Check sheet for the modelled part. Datum: model origin and axes. Units: mm. A direction names the side the tool comes from. Give positions to 0.01 mm unless a question says otherwise; leave off trailing zeros. Order: outer loops, then holes, each group sorted by start corner. A loop starts at its lowest first (then second) coordinate and runs counter-clockwise, first axis right, second up.
```python
from build123d import *

# Parameters (mm, degrees)
IZIM1_R                     = 6.55
Y_KSEKLIK_EKSTR_ZYON1_DEPTH = 1.6
IZIM2_R                     = 1.5
KES_EKSTR_ZYON1_DEPTH       = 1.6


with BuildPart() as part:
    # Çizim1 → Yükseklik-Ekstrüzyon1 (new body)
    with BuildSketch(Plane.XY):
        with BuildLine():
            Line((51.878679656, -0.878679656), (62.901413512, -11.901413512))
            ThreePointArc((62.901413512, -11.901413512), (63.179114484, -12.782168471), (62.616924992, -13.51482808))
            Line((62.616924992, -13.51482808), (61.615557944, -13.981773203))
            ThreePointArc((61.615557944, -13.981773203), (60.959512838, -14.047839782), (60.404952381, -13.691156907))
            ThreePointArc((60.404952381, -13.691156907), (53.799180994, -16.856750014), (61.123557768, -16.753308252))
            ThreePointArc((61.123557768, -16.753308252), (61.318334892, -16.334489822), (61.680554911, -16.047882666))
            Line((61.680554911, -16.047882666), (63.577381738, -15.16337779))
            ThreePointArc((63.577381738, -15.16337779), (64.537299608, -15.226294131), (65, -16.069685577))
            Line((65, -16.069685577), (65, -66.030314423))
            ThreePointArc((65, -66.030314423), (64.537299608, -66.873705869), (63.577381738, -66.93662221))
            Line((63.577381738, -66.93662221), (61.680554911, -66.052117334))
            ThreePointArc((61.680554911, -66.052117334), (61.318334892, -65.765510178), (61.123557768, -65.346691748))
            ThreePointArc((61.123557768, -65.346691748), (53.799180994, -65.243249986), (60.404952381, -68.408843093))
            ThreePointArc((60.404952381, -68.408843093), (60.959512838, -68.052160218), (61.615557944, -68.118226797))
            Line((61.615557944, -68.118226797), (62.616924992, -68.58517192))
            ThreePointArc((62.616924992, -68.58517192), (63.179114484, -69.317831529), (62.901413512, -70.198586488))
            Line((62.901413512, -70.198586488), (51.878679656, -81.221320344))
            ThreePointArc((51.878679656, -81.221320344), (50.90540961, -81.871638598), (49.757359313, -82.1))
            Line((49.757359313, -82.1), (34.45, -82.1))
            ThreePointArc((34.45, -82.1), (33.742893219, -81.807106781), (33.45, -81.1))
            Line((33.45, -81.1), (33.45, -80.681281566))
            ThreePointArc((33.45, -80.681281566), (33.610200525, -80.138384852), (34.039473684, -79.769432815))
            ThreePointArc((34.039473684, -79.769432815), (32.5, -72.6), (30.960526316, -79.769432815))
            ThreePointArc((30.960526316, -79.769432815), (31.389799475, -80.138384852), (31.55, -80.681281566))
            Line((31.55, -80.681281566), (31.55, -81.1))
            ThreePointArc((31.55, -81.1), (31.257106781, -81.807106781), (30.55, -82.1))
            Line((30.55, -82.1), (15.242640687, -82.1))
            ThreePointArc((15.242640687, -82.1), (14.09459039, -81.871638598), (13.121320344, -81.221320344))
            Line((13.121320344, -81.221320344), (2.098586488, -70.198586488))
            ThreePointArc((2.098586488, -70.198586488), (1.820885516, -69.317831529), (2.383075008, -68.58517192))
            Line((2.383075008, -68.58517192), (3.384442056, -68.118226797))
            ThreePointArc((3.384442056, -68.118226797), (4.040487162, -68.052160218), (4.595047619, -68.408843093))
            ThreePointArc((4.595047619, -68.408843093), (11.200819006, -65.243249986), (3.876442232, -65.346691748))
            ThreePointArc((3.876442232, -65.346691748), (3.681665108, -65.765510178), (3.319445089, -66.052117334))
            Line((3.319445089, -66.052117334), (1.422618262, -66.93662221))
            ThreePointArc((1.422618262, -66.93662221), (0.462700392, -66.873705869), (0, -66.030314423))
            Line((0, -66.030314423), (0, -16.069685577))
            ThreePointArc((0, -16.069685577), (0.462700392, -15.226294131), (1.422618262, -15.16337779))
            Line((1.422618262, -15.16337779), (3.319445089, -16.047882666))
            ThreePointArc((3.319445089, -16.047882666), (3.681665108, -16.334489822), (3.876442232, -16.753308252))
            ThreePointArc((3.876442232, -16.753308252), (11.200819006, -16.856750014), (4.595047619, -13.691156907))
            ThreePointArc((4.595047619, -13.691156907), (4.040487162, -14.047839782), (3.384442056, -13.981773203))
            Line((3.384442056, -13.981773203), (2.383075008, -13.51482808))
            ThreePointArc((2.383075008, -13.51482808), (1.820885516, -12.782168471), (2.098586488, -11.901413512))
            Line((2.098586488, -11.901413512), (13.121320344, -0.878679656))
            ThreePointArc((13.121320344, -0.878679656), (14.09459039, -0.228361402), (15.242640687, 0))
            Line((15.242640687, 0), (30.55, 0))
            ThreePointArc((30.55, 0), (31.257106781, -0.292893219), (31.55, -1))
            Line((31.55, -1), (31.55, -1.418718434))
            ThreePointArc((31.55, -1.418718434), (31.389799475, -1.961615148), (30.960526316, -2.330567185))
            ThreePointArc((30.960526316, -2.330567185), (32.5, -9.5), (34.039473684, -2.330567185))
            ThreePointArc((34.039473684, -2.330567185), (33.610200525, -1.961615148), (33.45, -1.418718434))
            Line((33.45, -1.418718434), (33.45, -1))
            ThreePointArc((33.45, -1), (33.742893219, -0.292893219), (34.45, 0))
            Line((34.45, 0), (49.757359313, 0))
            ThreePointArc((49.757359313, 0), (50.90540961, -0.228361402), (51.878679656, -0.878679656))
        make_face()
        with Locations((21.25, -11)):
            Circle(IZIM1_R, mode=Mode.SUBTRACT)
        with Locations((43.75, -11)):
            Circle(IZIM1_R, mode=Mode.SUBTRACT)
        with Locations(Location((43.75, -71.1, 0), (0, 0, 180))):
            Circle(IZIM1_R, mode=Mode.SUBTRACT)
        with Locations(Location((21.25, -71.1, 0), (0, 0, 180))):
            Circle(IZIM1_R, mode=Mode.SUBTRACT)
    extrude(amount=Y_KSEKLIK_EKSTR_ZYON1_DEPTH)

    # Çizim2 → Kes-Ekstrüzyon1 (cut)
    with BuildSketch(Plane.XY.offset(1.6)):
        with Locations((32.5, -41.05)):
            Circle(IZIM2_R)
    extrude(amount=-KES_EKSTR_ZYON1_DEPTH, mode=Mode.SUBTRACT)


solid = part.part
```
Q1. Tool access check on faces 1 (the cylindrical face through (14.079, -0.235, 0.789)), 2 (the flat face through (2.38, -66.49, 0.79)). Record the directions out of +Z, -Z, +X, -X, +Y, -Y that give a thin tool (end or side, any length) a straight path to the whole face; none if there is none.
Q2. Sectioned sample at C-C, the plane y = -11. Record the cut outline in (x, z).
Q3. Draft check along Y on faces 3 (the cylindrical face through (53.77, -16.72, 0.79)), 4 (the cylindrical face through (50.921, -81.865, 0.789)), 5 (the flat face through (42, 0, 1)). Enter one of: pulls with the +Y half, pulls with the -Y half, needs draft (parallel to the pull), parting line crosses it, or undercut.
Q4. Material ranges on line 1 (Y direction, x = 24, z = 0.8); line 2 (Y direction, x = 22.5, z = 0.35); line 3 (X direction, y = -5.75, z = 0.95), recorded low to high.
Q5. Sectioned sample at D-D, the plane y = -76.35. Record the cut outline in (x, z), plus the area to 3 significant figures.
Q6. Sectioned sample at B-B, the plane x = 7.55. Record the cut outline in (y, z), plus the area to 3 significant figures.
Q7. Sectioned sample at A-A, the plane y = -41.05. Record the cut outline in (x, z), plus the area to 3 significant figures.
Filled in:
1. face 1: +Z, -Z, -X, +Y
1. face 2: +Z, -Z
2. outline: (3, 0) - (14.7, 0) - (14.7, 1.6) - (3, 1.6) - close; (27.8, 0) - (37.2, 0) - (37.2, 1.6) - (27.8, 1.6) - close; (50.3, 0) - (62, 0) - (62, 1.6) - (50.3, 1.6) - close
3. face 3: undercut
3. face 4: pulls with the -Y half
3. face 5: pulls with the +Y half
4. line 1: y = -82.1 to -77.04, -65.16 to -16.94, -5.06 to 0
4. line 2: y = -82.1 to -77.53, -64.67 to -17.43, -4.57 to 0
4. line 3: x = 8.25 to 17.33, 25.17 to 28.75, 36.25 to 39.83, 47.67 to 56.75
5. outline: (8.25, 0) - (17.33, 0) - (17.33, 1.6) - (8.25, 1.6) - close; (25.17, 0) - (28.75, 0) - (28.75, 1.6) - (25.17, 1.6) - close; (36.25, 0) - (39.83, 0) - (39.83, 1.6) - (36.25, 1.6) - close; (47.67, 0) - (56.75, 0) - (56.75, 1.6) - (47.67, 1.6) - close
5. area: 40.5 mm2
6. outline: (-75.65, 0) - (-69.85, 0) - (-69.85, 1.6) - (-75.65, 1.6) - close; (-62.35, 0) - (-19.75, 0) - (-19.75, 1.6) - (-62.35, 1.6) - close; (-12.25, 0) - (-6.45, 0) - (-6.45, 1.6) - (-12.25, 1.6) - close
6. area: 86.7 mm2
7. outline: (0, 0) - (31, 0) - (31, 1.6) - (0, 1.6) - close; (34, 0) - (65, 0) - (65, 1.6) - (34, 1.6) - close
7. area: 99.2 mm2
